Source: CAD feature listing. Evaluate the final solid. Frame: model axes, mm. Give positions to 0.01 mm unless a question says otherwise; leave off trailing zeros.
1) Material intervals for line 1 (Y direction, x = -137.5, z = 352), sorted ascending.
2) First-contact query: P1, Ø4.5, axis at x = 4, z = -387.5, coming from the +Y side. Flat tip, straight axial feed; report the tip coordinate or a pass-through.
3) Section A-A, the plane y = -2.5. Give the number of separate pieces and of enclosed holes in the cut face, plus the area to 3 significant figures.
```python
from build123d import *

# Parameters (mm, degrees)
F0_W     = 400
F0_H     = 1000
F2_DEPTH = 12
F1_W     = 400
F1_H     = 9
F3_DEPTH = 5


with BuildPart() as f2:
    # F0 (on Front) → F2 (new body)
    with BuildSketch(Plane.XZ):
        Rectangle(F0_W, F0_H)
    extrude(amount=F2_DEPTH)

    # F1 (on face) → F3 (cut)
    with BuildSketch(Plane.XZ):
        with Locations((0, -483.5)):
            Rectangle(F1_W, F1_H)
        with Locations((0, -434.5)):
            Rectangle(F1_W, F1_H)
        with Locations((0, -385.5)):
            Rectangle(F1_W, F1_H)
        with Locations((0, -336.5)):
            Rectangle(F1_W, F1_H)
        with Locations((0, -287.5)):
            Rectangle(F1_W, F1_H)
        with Locations((0, -238.5)):
            Rectangle(F1_W, F1_H)
        with Locations((0, -189.5)):
            Rectangle(F1_W, F1_H)
        with Locations((0, -140.5)):
            Rectangle(F1_W, F1_H)
        with Locations((0, -91.5)):
            Rectangle(F1_W, F1_H)
        with Locations((0, -42.5)):
            Rectangle(F1_W, F1_H)
        with Locations((0, 6.5)):
            Rectangle(F1_W, F1_H)
        with Locations((0, 55.5)):
            Rectangle(F1_W, F1_H)
        with Locations((0, 104.5)):
            Rectangle(F1_W, F1_H)
        with Locations((0, 153.5)):
            Rectangle(F1_W, F1_H)
        with Locations((0, 202.5)):
            Rectangle(F1_W, F1_H)
        with Locations((0, 251.5)):
            Rectangle(F1_W, F1_H)
        with Locations((0, 300.5)):
            Rectangle(F1_W, F1_H)
        with Locations((0, 349.5)):
            Rectangle(F1_W, F1_H)
        with Locations((0, 398.5)):
            Rectangle(F1_W, F1_H)
        with Locations((0, 447.5)):
            Rectangle(F1_W, F1_H)
    extrude(amount=F3_DEPTH, mode=Mode.SUBTRACT)


solid = f2.part
```
From the geometry:
1. line 1: y = -12 to -5
2. P1: stops at y = -5
3. separate pieces: 21
3. enclosed holes: 0
3. area: 328,000 mm2
